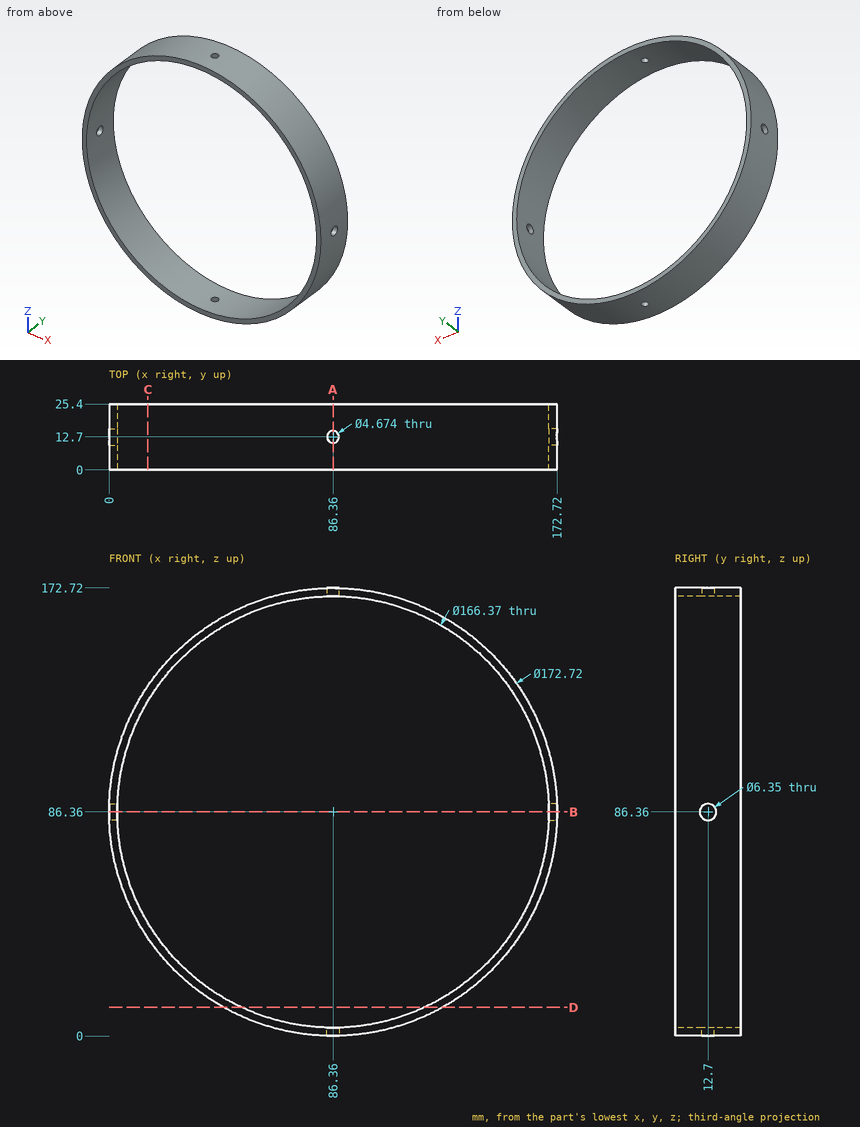
For this review, use the dimensioned drawing (mm, ordinates from the lowest corner) and the shaded views. Round coordinates to 2 decimals unless told otherwise and drop trailing zeros. Write each loop counter-clockwise with the first axis right and the second up, starting at its lowest first coordinate (ties: lowest second). Pieces come first, ordered by that corner, then holes. Notation, with made-up numbers: (55, 76.25) - (72, 76.25) arc R34 ccw to (72, 109.25) - close; hole circle Ø8 at (-0.5, -23). An arc over 180 degrees is marked (long way). Answer as a JSON object with one key per item and string values.
1. For pin 1 Ø1 at (x, y) = (108, 19) entering from -Z; pin 2 Ø2 at (y, z) = (7, 98) entering from -X; pin 3 Ø3 at (y, z) = (12.5, 128.5) entering from +X, all flat-tipped, find the tip position at first contact; note any pin that passes through.
Response values:
{"pin 1": "stops at z = 2.63", "pin 2": "stops at x = 0.66", "pin 3": "stops at x = 162.56"}
2. We need section A-A on x = 86.36. Give the boundary of the cut face in (y, z) (1 decimal).
Response values:
{"outline": "(0, 0) - (10.4, 0) - (10.4, 3.2) - (0, 3.2) - close; (0, 169.5) - (10.4, 169.5) - (10.4, 172.7) - (0, 172.7) - close; (15, 0) - (25.4, 0) - (25.4, 3.2) - (15, 3.2) - close; (15, 169.5) - (25.4, 169.5) - (25.4, 172.7) - (15, 172.7) - close"}
3. We need section B-B on z = 86.36. Give the boundary of the cut face in (x, y) (1 decimal).
Response values:
{"outline": "(0, 0) - (3.2, 0) - (3.2, 9.5) - (0, 9.5) - close; (0, 15.9) - (3.2, 15.9) - (3.2, 25.4) - (0, 25.4) - close; (169.5, 0) - (172.7, 0) - (172.7, 9.5) - (169.5, 9.5) - close; (169.5, 15.9) - (172.7, 15.9) - (172.7, 25.4) - (169.5, 25.4) - close"}
4. To check wall thickness, follow line 1 along Z through (x, y) = (89, 21.25); line 2 along X through (y, z) = (21, 96.5) (1 decimal); line 3 along Z through (x, y) = (64, 2) (1 decimal). State the ranges of each line that lie inside material, in increasing order.
Response values:
{"line 1": "z = 0.04 to 3.22, 169.5 to 172.68", "line 2": "x = 0.6 to 3.8, 168.9 to 172.1", "line 3": "z = 2.9 to 6.2, 166.5 to 169.8"}
5. We need section C-C on x = 15. Give the boundary of the cut face in (y, z).
Response values:
{"outline": "(0, 37.72) - (25.4, 37.72) - (25.4, 43.61) - (0, 43.61) - close; (0, 129.11) - (25.4, 129.11) - (25.4, 135) - (0, 135) - close"}
6. We need section D-D on z = 11. Give the boundary of the cut face in (x, y).
Response values:
{"outline": "(44.18, 0) - (51.14, 0) - (51.14, 25.4) - (44.18, 25.4) - close; (121.58, 0) - (128.54, 0) - (128.54, 25.4) - (121.58, 25.4) - close"}
